Design review of the part built by this model. Coordinates are the model's own, in mm. Face numbers are marked on the shaded views. Give positions to 0.01 mm unless a question says otherwise; leave off trailing zeros. Loops run counter-clockwise (first coordinate to the right, second up) from the corner with the lowest first, then second, coordinate; pieces in that order, holes last.
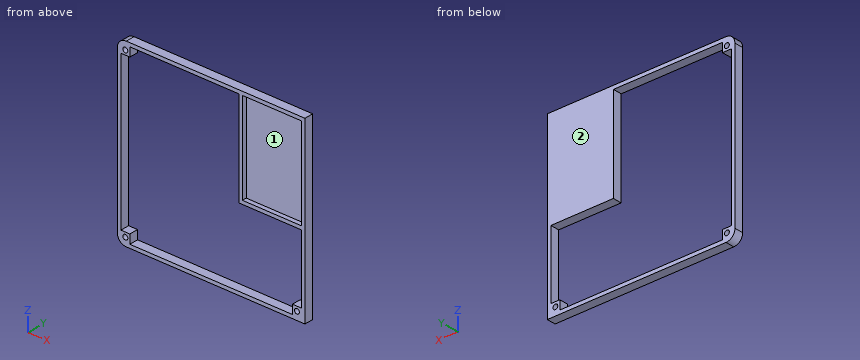
from build123d import *

# Parameters (mm, degrees)
SKETCH1_W                = 210
SKETCH1_H                = 200
SKETCH1_W_2              = 202
SKETCH1_H_2              = 192
BOSS_EXTRUDE1_DEPTH      = 10
SKETCH2_W                = 70
SKETCH2_H                = 106
BOSS_EXTRUDE2_DEPTH      = 10
SKETCH3_W                = 66
SKETCH3_H                = 102
CUT_EXTRUDE1_DEPTH       = 5
SKETCH4_W                = 10
SKETCH4_H                = 10
SKETCH4_R                = 2.75
BOSS_EXTRUDE3_DEPTH      = 10
FILLET1_R                = 10
BOSS_EXTRUDE4_DEPTH      = 5
BOSS_EXTRUDE4_DEPTH_BACK = 5


with BuildPart() as part:
    # Sketch1 → Boss-Extrude1 (new body)
    with BuildSketch(Plane(origin=(0, 0, 0), x_dir=(1, 0, 0), z_dir=(0, 1, 0))):
        with Locations((105, 100)):
            Rectangle(SKETCH1_W, SKETCH1_H)
        with Locations((105, 100)):
            Rectangle(SKETCH1_W_2, SKETCH1_H_2, mode=Mode.SUBTRACT)
    extrude(amount=-BOSS_EXTRUDE1_DEPTH)

    # Sketch2 → Boss-Extrude2 (add)
    with BuildSketch(Plane.XZ.offset(10)):
        with Locations((175, -53)):
            Rectangle(SKETCH2_W, SKETCH2_H)
    extrude(amount=-BOSS_EXTRUDE2_DEPTH)

    # Sketch3 → Cut-Extrude1 (cut)
    with BuildSketch(Plane.XZ.offset(10)):
        with Locations((173, -55)):
            Rectangle(SKETCH3_W, SKETCH3_H)
    extrude(amount=-CUT_EXTRUDE1_DEPTH, mode=Mode.SUBTRACT)

    # Sketch4 → Boss-Extrude3 (add)
    with BuildSketch(Plane.XZ.offset(10)):
        with Locations((9, -9)):
            Rectangle(SKETCH4_W, SKETCH4_H)
        with Locations((9, -9)):
            Circle(SKETCH4_R, mode=Mode.SUBTRACT)
        with Locations((9, -191)):
            Rectangle(SKETCH4_W, SKETCH4_H)
        with Locations((9, -191)):
            Circle(SKETCH4_R, mode=Mode.SUBTRACT)
        with Locations((201, -191)):
            Rectangle(SKETCH4_W, SKETCH4_H)
        with Locations((201, -191)):
            Circle(SKETCH4_R, mode=Mode.SUBTRACT)
    extrude(amount=-BOSS_EXTRUDE3_DEPTH)

    # Fillet1
    fillet1_edges = [part.edges().sort_by_distance(p)[0] for p in [
        (0, -5, -200),
        (0, -5, 0),
    ]]
    fillet(fillet1_edges, radius=FILLET1_R)

    # Sketch5 → Boss-Extrude4 (add, two sides)
    with BuildSketch(Plane.XZ.offset(5)) as boss_extrude4_sk:
        Polygon((206, -110), (206, -106), (140, -106), (140, -4), (136, -4), (136, -110), align=None)
    extrude(amount=BOSS_EXTRUDE4_DEPTH)
    extrude(boss_extrude4_sk.sketch, amount=-BOSS_EXTRUDE4_DEPTH_BACK)


solid = part.part
Q1. Take a section at D-D (x = 162.5). Give the boundary of the cut face in (y, z), plus the area to 3 significant figures.
Results:
outline: (-10, -200) - (0, -200) - (0, -196) - (-10, -196) - close; (-10, -110) - (0, -110) - (0, 0) - (-10, 0) - (-10, -4) - (-5, -4) - (-5, -106) - (-10, -106) - close
area: 630 mm2
Q2. Take a section at C-C (y = -6.5). Give the boundary of the cut face in (x, z).
Results:
outline: (0, -190) arc R10 ccw to (10, -200) - (210, -200) - (210, 0) - (10, 0) arc R10 ccw to (0, -10) - close; hole (4, -186) - (14, -186) - (14, -196) - (196, -196) - (196, -186) - (206, -186) - (206, -110) - (136, -110) - (136, -4) - (14, -4) - (14, -14) - (4, -14) - close; hole circle Ø5.5 at (9, -191); hole circle Ø5.5 at (9, -9); hole (140, -106) - (206, -106) - (206, -4) - (140, -4) - close; hole circle Ø5.5 at (201, -191)
Q3. Take a section at A-A (z = -87.5). Give the boundary of the cut face in (x, y).
Results:
outline: (0, -10) - (4, -10) - (4, 0) - (0, 0) - close; (136, -10) - (140, -10) - (140, -5) - (206, -5) - (206, -10) - (210, -10) - (210, 0) - (136, 0) - close
Q4. Draft analysis for pull direction X (two halves, no side actions). For the marked faces 1 and 2, state which applies: pulls with the +X half, pulls with the -X half, needs draft (parallel to the pull), parting line crosses it, or undercut.
Results:
face 1: undercut
face 2: needs draft
Q5. Wall thickness on line 1 (X direction, y = -6, z = -80); line 2 (Z direction, x = 9, y = -6.5); line 3 (X direction, y = -3, z = -191): over which ranges is each line inside the solid? List them lowest first.
Results:
line 1: x = 0 to 4, 136 to 140, 206 to 210
line 2: z = -199.95 to -193.75, -188.25 to -186, -14 to -11.75, -6.25 to -0.05
line 3: x = 0.05 to 6.25, 11.75 to 14, 196 to 198.25, 203.75 to 210
Q6. Insertion check: pin 1 (4 mm diameter, centred on x = 184.5, z = -81.5, fed in from +Y). The pin has a flat end and moves straight along its axis. Give the tip position at first contact, or say it passes through.
Results:
pin 1: stops at y = 0
Q7. Take a section at B-B (x = 201). Give the boundary of the cut face in (y, z), plus the area to 3 significant figures.
Results:
outline: (-10, -200) - (0, -200) - (0, -193.75) - (-10, -193.75) - close; (-10, -188.25) - (0, -188.25) - (0, -186) - (-10, -186) - close; (-10, -110) - (0, -110) - (0, 0) - (-10, 0) - (-10, -4) - (-5, -4) - (-5, -106) - (-10, -106) - close
area: 675 mm2
